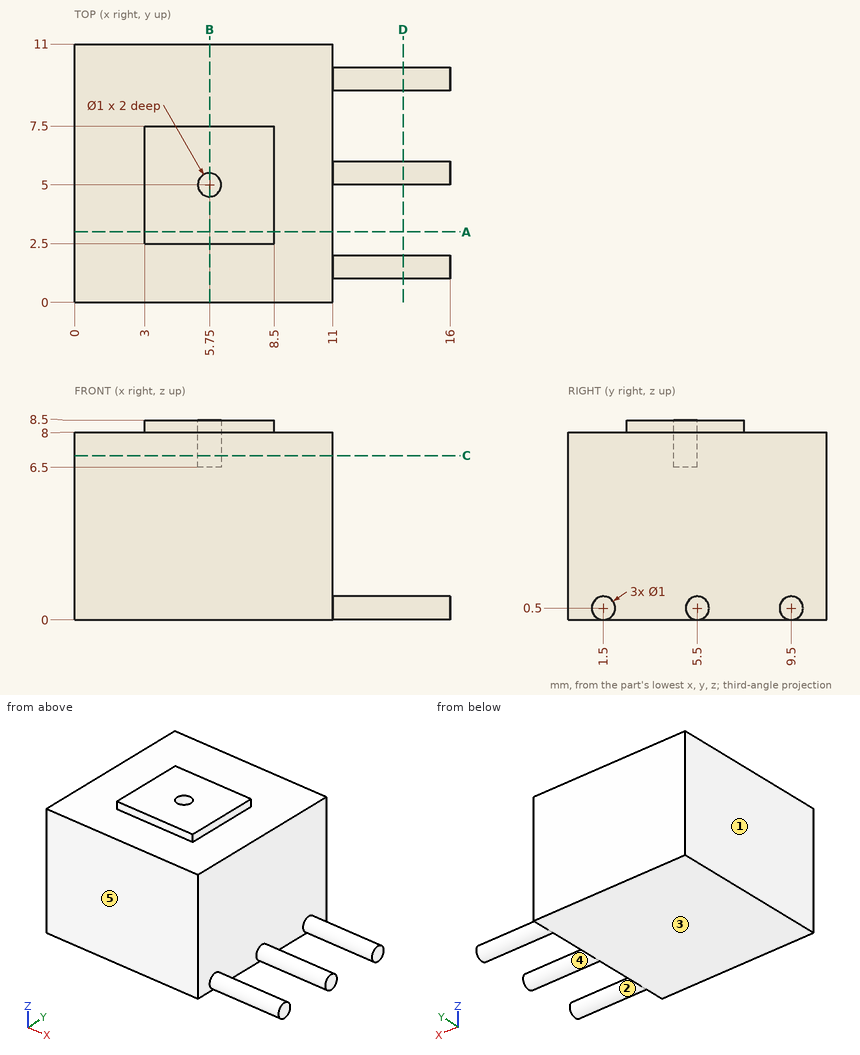
Here's the drawing with two shaded views (mm, measured from the low corner). I have some questions. A direction names the side the tool comes from. Round coordinates to 2 decimals unless told otherwise and drop trailing zeros. Write each loop counter-clockwise with the first axis right and the second up, starting at its lowest first coordinate (ties: lowest second). Pieces come first, ordered by that corner, then holes.
(1) Suppose I cut it at C-C on z = 7. Write out the boundary of the cut face in (x, y).
Findings below:
outline: (0, 0) - (11, 0) - (11, 11) - (0, 11) - close; hole circle Ø1 at (5.75, 5)
(2) Which directions (+Z, -Z, +X, -X, +Y, -Y) give clear straight access to the entire face, cutting with the end or side of a thin tool? Please do the marked faces 1 and 2.
Findings below:
face 1: +Z, -Z, -X, +Y, -Y
face 2: +X
(3) Thinking about a two-plate mould opening in Y: for the marked faces 3, 4 and 5, which applies, +Y half, -Y half, draft (parallel to the pull), parting line (faces both ways), or undercut?
Findings below:
face 3: draft
face 4: undercut
face 5: -Y half
(4) If I drill on probe 1 along Y at (x, z) = (5.75, 7.9); probe 2 along X at (y, z) = (3.5, 5.25); probe 3 along Z at (x, y) = (2, 9), over which ranges is the centre line in solid material (lowest first)?
Findings below:
probe 1: y = 0 to 4.5, 5.5 to 11
probe 2: x = 0 to 11
probe 3: z = 0 to 8
(5) Suppose I cut it at D-D on x = 14. Write out the boundary of the cut face in (y, z).
Findings below:
outline: circle Ø1 at (1.5, 0.5); circle Ø1 at (5.5, 0.5); circle Ø1 at (9.5, 0.5)
(6) Suppose I cut it at A-A on y = 3. Write out the boundary of the cut face in (x, z).
Findings below:
outline: (0, 0) - (11, 0) - (11, 8) - (8.5, 8) - (8.5, 8.5) - (3, 8.5) - (3, 8) - (0, 8) - close
(7) For pin 1 (2 mm diameter, centred on y = 8, z = 4, fed in from +X); pin 2 (5 mm diameter, centred on x = 11.5, y = 5, fed in from +Z), each with a flat end and sliding along its axis, tell me the tip position at first contact or that it passes through.
Findings below:
pin 1: stops at x = 11
pin 2: stops at z = 8
(8) Suppose I cut it at B-B on x = 5.75. Write out the boundary of the cut face in (y, z), and give its area (3 significant figures).
Findings below:
outline: (0, 0) - (11, 0) - (11, 8) - (7.5, 8) - (7.5, 8.5) - (5.5, 8.5) - (5.5, 6.5) - (4.5, 6.5) - (4.5, 8.5) - (2.5, 8.5) - (2.5, 8) - (0, 8) - close
area: 88.5 mm2
